Input: part model. Units: mm. Frame: model coordinates. Face numbers are marked on the shaded views. A direction names the side the tool comes from. Give positions to 0.01 mm unless a question says otherwise; leave off trailing zeros. Loops run counter-clockwise (first coordinate to the right, second up) from the corner with the lowest first, then second, coordinate; pieces in that order, holes last. Notation, with made-up numbers: M 11.5,22 L 57.5,22 A32 ccw 57.5,61 Z; hole C 78.5,-39 d10. An arc over 180 degrees is marked long. One line per item, written item: value. Start each with the question number.
(1) Pull-direction query (Z, two-part tool) for the marked faces 1, 2, 3 and 4; classes: released by +Z, released by -Z, zero draft, split by the parting line, or undercut.
(2) Ray query, line 1 along Z through (x, y) = (-5, -5); line 2 along X through (y, z) = (-9.5, -12.5). Return the intervals inside material, ascending. Write a range as from..to.
(3) Section C-C on y = -18.5. Output: boundary loops of the cut face in (x, z), plus the area to 3 significant figures.
(4) Section A-A on z = -6. Output: boundary loops of the cut face in (x, y), plus the area to 3 significant figures.
(5) Access query for the marked faces 5 and 6. Directions: +Z, -Z, +X, -X, +Y, -Y. A direction counts if a zero-diameter tool reaches every point of the face in a straight line with its end or side. Return the directions, or none.
(6) Pin query (flat end, axial travel): P1, Ø1, axis at y = -5.5, z = -15, coming from the +X side; P2, Ø12, axis at x = 15.5, y = -11, coming from the -Z side. Return the tip coordinate at first contact, or that it passes through.
(7) Section B-B on x = -7.5. Output: boundary loops of the cut face in (y, z), plus the area to 3 significant figures.
(8) Section D-D on x = 17. Output: boundary loops of the cut face in (y, z).
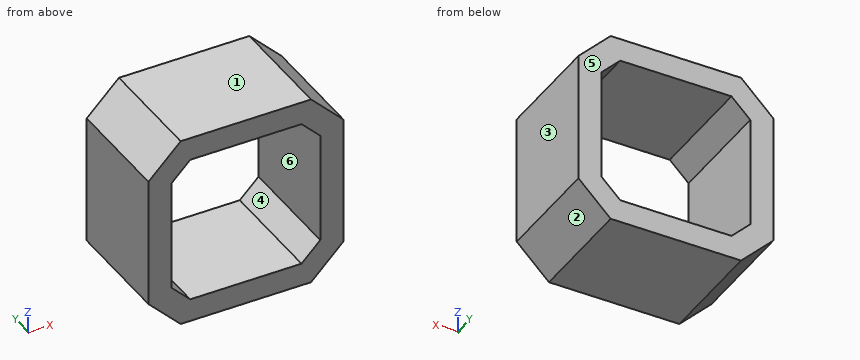
```python
from build123d import *

# Parameters (mm, degrees)
F1_DEPTH = 24
F3_DEPTH = 24.001


with BuildPart() as f1:
    # F0 (on Front) → F1 (new body)
    with BuildSketch(Plane.XZ):
        Polygon((21.15, 14.15), (14.15, 21.15), (-14.15, 21.15), (-21.15, 14.15), (-21.15, -14.15), (-14.15, -21.15), (14.15, -21.15), (21.15, -14.15), align=None)
    extrude(amount=F1_DEPTH)

    # F2 (on face) → F3 (cut, through all)
    with BuildSketch(Plane.XZ.offset(24)):
        Polygon((12.078932, -16.15), (16.15, -12.078932), (16.15, 12.078932), (12.078932, 16.15), (-12.078932, 16.15), (-16.15, 12.078932), (-16.15, -12.078932), (-12.078932, -16.15), align=None)
    extrude(amount=-F3_DEPTH, mode=Mode.SUBTRACT)


solid = f1.part
```
Output values:
1. face 1: released by +Z
1. face 2: released by -Z
1. face 3: zero draft
1. face 4: undercut
2. line 1: z = -21.15..-16.15, 16.15..21.15
2. line 2: x = -21.15..-15.73, 15.73..21.15
3. outline: M -21.15,-14.15 L -14.15,-21.15 L 14.15,-21.15 L 21.15,-14.15 L 21.15,14.15 L 14.15,21.15 L -14.15,21.15 L -21.15,14.15 Z; hole M -16.15,-12.08 L -12.08,-16.15 L 12.08,-16.15 L 16.15,-12.08 L 16.15,12.08 L 12.08,16.15 L -12.08,16.15 L -16.15,12.08 Z
3. area: 681 mm²
4. outline: M -21.15,-24 L -16.15,-24 L -16.15,0 L -21.15,0 Z; M 16.15,-24 L 21.15,-24 L 21.15,0 L 16.15,0 Z
4. area: 240 mm²
5. face 5: +Z, -Z, +X, -X, +Y
5. face 6: +Y, -Y
6. P1: stops at x = 20.8
6. P2: stops at z = -21.15
7. outline: M -24,-21.15 L 0,-21.15 L 0,-16.15 L -24,-16.15 Z; M -24,16.15 L 0,16.15 L 0,21.15 L -24,21.15 Z
7. area: 240 mm²
8. outline: M -24,-18.3 L 0,-18.3 L 0,18.3 L -24,18.3 Z
